Here's how the part is built. I have some questions about the finished solid (model axes, mm). Face numbers are marked on the shaded views. Round coordinates to 2 decimals unless told otherwise and drop trailing zeros. Loops run counter-clockwise (first coordinate to the right, second up) from the corner with the lowest first, then second, coordinate; pieces in that order, holes last. Notation, with made-up numbers: M -15,-24 L 33,-24 A25 cw 33,-10 Z; hole C 5,78.25 d9. An arc over 180 degrees is marked long. Put each result on its own line as item: value. Start each with the question number.
Autodesk Inventor part; units mm, degrees
ref_plane "YZ Plane" through (0, 0, 0) normal (1, 0, 0) x (0, 1, 0)
ref_plane "XZ Plane" through (0, 0, 0) normal (0, 1, 0) x (-1, 0, 0)
ref_plane "XY Plane" through (0, 0, 0) normal (0, 0, 1) x (1, 0, 0)
sketch "Sketch1" plane through (0, 0, 0) normal (0, 0, 1) x (1, 0, 0)
  line L0 (-43.75, 33) -> (43.75, 33)
  line L1 (43.75, 33) -> (43.75, -33)
  line L2 (43.75, -33) -> (-43.75, -33)
  line L3 (-43.75, -33) -> (-43.75, 33)
  point P0 (0, 0)
  point P1 (0, 33)
  point P2 (-43.75, 0)
  dimension "d0" = 87.5
  dimension "d1" = 66
extrude "Extrusion1" add sketch "Sketch1" along normal blind 8
sketch "Sketch4" plane through (0, 0, 8) normal (0, 0, 1) x (1, 0, 0)
  line L0 (43.75, 33) -> (-43.75, 33)
  line L1 (-43.75, 33) -> (-43.75, -33)
  circle A0 centre (-35.25, 24) radius 5.4
  circle A1 centre (-35.25, -24) radius 5.4
  line L2 (-43.75, -33) -> (43.75, -33)
  point P0 (0, 0)
  dimension "d27" = 8.5
  dimension "d28" = 9
  dimension "d29" = 10.8
  dimension "d30" = 9
extrude "Extrusion4" cut sketch "Sketch4" against normal through all
sketch "Sketch5" plane through (0, 0, 8) normal (0, 0, 1) x (1, 0, 0)
  circle A0 centre (-23.0012, 0) radius 4
  circle A1 centre (-23.0012, 0) radius 8
  line L0 (-43.75, 33) -> (-43.75, -33)
  line L1 (43.75, 33) -> (-43.75, 33)
  circle A2 centre (-23.0012, 0) radius 7
  point P0 (0, 0)
  point P1 (-43.75, 0)
  dimension "d24" = 16
  dimension "d33" = 20.7488
extrude "Extrusion5" cut sketch "Sketch5" against normal through all contours A0 | A1 | A2
sketch "Sketch6" plane through (0, 0, 8) normal (0, 0, 1) x (1, 0, 0)
  circle A0 centre (-33.7512, 10) radius 1.75
  circle A1 centre (-12.2512, 10) radius 1.75
  circle A2 centre (-12.2512, -10) radius 1.75
  circle A3 centre (-33.7512, -10) radius 1.75
  line L0 (-33.7512, 10) -> (-12.2512, 10)
  line L1 (-12.2512, 10) -> (-12.2512, -10)
  line L2 (-12.2512, -10) -> (-33.7512, -10)
  line L3 (-33.7512, -10) -> (-33.7512, 10)
  line L4 (-33.7512, 10) -> (-12.2512, -10) construction
  line L5 (-12.2512, 10) -> (-33.7512, -10) construction
  circle A4 centre (-23.0012, 0) radius 8
  line L6 (-43.75, 33) -> (-43.75, -33)
  point P0 (0, 0)
  point P1 (-23.0012, 0)
  dimension "d35" = 3.5
  dimension "d36" = 21.5
  dimension "d37" = 20
extrude "Extrusion6" cut sketch "Sketch6" against normal through all contours L0 L3 A0 | A0 L3 L0 | L0 L1 A1 | A1 L1 L0 | L3 L2 A3 | A3 L2 L3 | L1 L2 A2 | A2 L2 L1
sketch "Sketch7" plane through (0, 0, 8) normal (0, 0, 1) x (1, 0, 0)
  point P0 (0, 0)
sketch "Sketch8" plane through (0, 0, 0) normal (0, 0, -1) x (-1, 0, 0)
  line L0 (-35.75, -33) -> (-43.75, -33)
  line L1 (-43.75, -33) -> (-43.75, 33)
  line L2 (-43.75, 33) -> (-35.75, 33)
  line L3 (-35.75, 33) -> (-35.75, -33)
  line L4 (-8.75, -33) -> (-16.75, -33)
  line L5 (-16.75, -33) -> (-16.75, 33)
  line L6 (-16.75, 33) -> (-8.75, 33)
  line L7 (-8.75, 33) -> (-8.75, -33)
  line L8 (-44.55, -20.5) -> (-44.55, -29.5)
  point P0 (0, 0)
  point P1 (-39.75, -28)
  point P2 (-39.75, -13)
  point P3 (-39.75, 13)
  point P4 (-39.75, 28)
  dimension "d38" = 4
  dimension "d39" = 5
  dimension "d40" = 15
  dimension "d41" = 5
  dimension "d42" = 15
  dimension "d56" = 26
hole "Hole1" at (39.75, 28, 0) direction (0, 0, 1) diameter 3.5 end through all
move faces "Move1" translate (2, 0, 0) faces at (43.75, -11, 2.6667)
pattern_linear "Rectangular Pattern2" count 2 spacing 15 along (0, -1, 0) count 2 spacing 41 along (0, -1, 0) of "Hole1"
pattern_linear "Rectangular Pattern3" count 2 spacing 27 along (-1, 0, 0) of "Hole1", "Rectangular Pattern2"
sketch "Sketch10" plane through (-43.75, 33, 8) normal (0, 1, 0) x (1, 0, 0)
  line L0 (0, 8) -> (0, 0)
  point P0 (43.75, 8)
  point P1 (8.5, 4)
  point P2 (0, 4)
  dimension "d66" = 8.5
hole "Hole2" at (-35.25, 33, 4) direction (0, -1, 0) diameter 4.134 depth 7.45 tip angle 118
sketch "Sketch11" plane through (-43.75, -33, 0) normal (0, -1, 0) x (1, 0, 0)
  line L0 (0, 0) -> (0, 8)
  point P0 (43.75, 0)
  point P1 (8.5, 4)
  point P2 (0, 4)
  dimension "d74" = 8.5
hole "Hole3" at (-35.25, -33, 4) direction (0, 1, 0) diameter 4.134 depth 7.45 tip angle 118
equation "\"d30\" = d28"
properties part number "0005-10-011" material "Wood (Maple)"
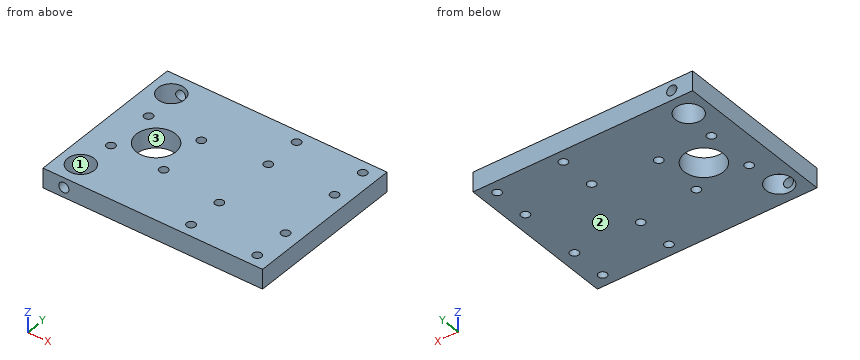
1) Suppose I cut it at C-C (y = 10). Write out the boundary of the cut face in (x, z), plus the area to 3 significant figures.
2) If I drill on probe 1 along Y at (x, z) = (39.75, 3.75); probe 2 along X at (y, z) = (13, 2); probe 3 along X at (y, z) = (-28, 5.5), over which ranges is the centre line in solid material (lowest first)? Write a range as from..to.
3) Suppose I cut it at D-D (z = 3). State how many separate pieces and enclosed holes the cut face has, plus the area to 3 significant figures.
4) I'm going to push flat-ended pins straight in: P1, Ø3.5, axis at x = -35.25, z = 4, coming from the +Y side; P2, Ø2, axis at x = -12.25, y = 10, coming from the +Z side; P3, Ø2.5, axis at x = -35.25, z = 4, coming from the +Y side. Where does each tip first touch, or does it pass through?
5) Suppose I cut it at A-A (y = 24). Write out the boundary of the cut face in (x, z).
6) If we mould it in two halves opening along X, with no side actions, what happens to the marked faces 1, 2 and 3? For each: pulls with the +X half, pulls with the -X half, needs draft (parallel to the pull), parting line crosses it, or undercut.
7) Suppose I cut it at B-B (x = 39.75). Write out the boundary of the cut face in (y, z), plus the area to 3 significant figures.
Results are:
1. outline: M -43.75,0 L -35.5,0 L -35.5,8 L -43.75,8 Z; M -32,0 L -14,0 L -14,8 L -32,8 Z; M -10.5,0 L 45.75,0 L 45.75,8 L -10.5,8 Z
1. area: 660 mm²
2. probe 1: -33..-29.75, -26.25..-14.75, -11.25..11.25, 14.75..26.25, 29.75..33
2. probe 2: -43.75..11, 14.5..38, 41.5..45.75
2. probe 3: -43.75..-38.88, -31.62..11, 14.5..38, 41.5..45.75
3. separate pieces: 1
3. enclosed holes: 13
3. area: 5,380 mm²
4. P1: y = 18.89
4. P2: through
4. P3: y = 18.75
5. outline: M -43.75,0 L -40.65,0 L -40.65,8 L -43.75,8 Z; M -29.85,0 L 45.75,0 L 45.75,8 L -29.85,8 Z
6. face 1: undercut
6. face 2: needs draft
6. face 3: undercut
7. outline: M -33,0 L -29.75,0 L -29.75,8 L -33,8 Z; M -26.25,0 L -14.75,0 L -14.75,8 L -26.25,8 Z; M -11.25,0 L 11.25,0 L 11.25,8 L -11.25,8 Z; M 14.75,0 L 26.25,0 L 26.25,8 L 14.75,8 Z; M 29.75,0 L 33,0 L 33,8 L 29.75,8 Z
7. area: 416 mm²
